```python
from build123d import *

# Parameters (mm, degrees)
SKETCH1_R           = 6.6675
BOSS_EXTRUDE1_DEPTH = 9.525
SKETCH3_R           = 6.6675
BOSS_EXTRUDE2_DEPTH = 9.525
BOSS_EXTRUDE2_TAPER = 9


with BuildPart() as part:
    # Sketch1 → Boss-Extrude1 (new, symmetric)
    with BuildSketch(Plane(origin=(0, 0, 0), x_dir=(0, 0, -1), z_dir=(1, 0, 0))):
        with Locations(Location((0, 0, 0), (0, 0, 180))):
            Circle(SKETCH1_R)
    extrude(amount=BOSS_EXTRUDE1_DEPTH, both=True)

    # Sketch3 → Boss-Extrude2 (add)
    with BuildSketch(Plane(origin=(9.525, 0, 0), x_dir=(0, 0, -1), z_dir=(1, 0, 0))):
        with Locations(Location((0, 0, 0), (0, 0, 180))):
            Circle(SKETCH3_R)
    boss_extrude2 = extrude(amount=BOSS_EXTRUDE2_DEPTH, taper=BOSS_EXTRUDE2_TAPER)

    # Mirror1: Boss-Extrude2 across plane
    add(boss_extrude2.mirror(Plane(origin=(0, 0, 0), x_dir=(0, 0, 1), z_dir=(1, 0, 0))))


solid = part.part
```
The model under review builds one solid part; all positions refer to its coordinate system, in mm. Round coordinates to 2 decimals unless told otherwise and drop trailing zeros. Loops run counter-clockwise (first coordinate to the right, second up) from the corner with the lowest first, then second, coordinate; pieces in that order, holes last.
1) Consider section B-B on x = -8. State the section outline as (y, z) points (1 decimal), then the cut area to 3 significant figures.
Values follow:
outline: circle Ø13.3 at (0, 0)
area: 140 mm2
2) Wall thickness on line 1 along Z through (x, y) = (-15.5, -1); line 2 along Z through (x, y) = (1.5, 5.5); line 3 along Y through (x, z) = (17, 0.75): over which ranges is each line inside the solid? List them lowest first.
Values follow:
line 1: z = -5.63 to 5.63
line 2: z = -3.77 to 3.77
line 3: y = -5.43 to 5.43
3) Clearance check with flat-ended pins moving along their axes: P1, Ø6, axis at x = 14.5, y = -4.5, coming from the -Z side; P2, Ø1, axis at x = 8.5, z = 4, coming from the +Y side (3 decimals); P3, Ø1, axis at x = -5.5, y = 4, coming from the +Z side (3 decimals). State where each tip first meets the part, or that it passes through.
Values follow:
P1: stops at z = -5.82
P2: stops at y = 5.675
P3: stops at z = 5.675
